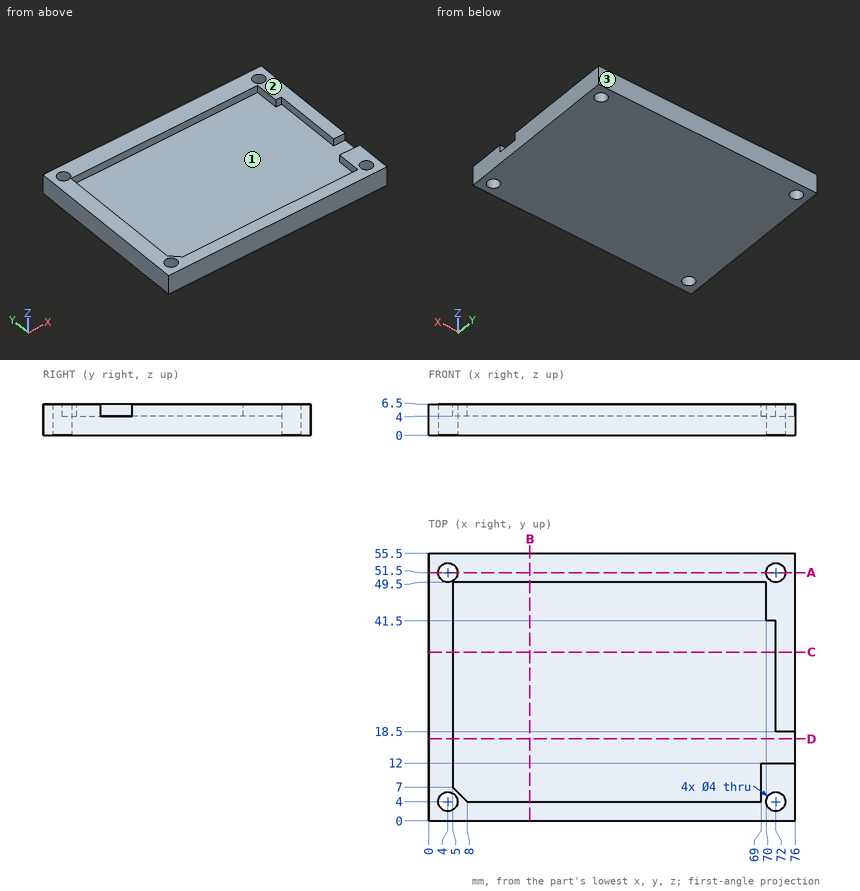
Could you check a few things on this drawing? It's one solid part, dimensions in mm from its lowest x, y, z. Give positions to 0.01 mm unless a question says otherwise; leave off trailing zeros. Write each loop counter-clockwise with the first axis right and the second up, starting at its lowest first coordinate (ties: lowest second). Pieces come first, ordered by that corner, then holes. Notation, with made-up numbers: M -26.75,-1 L -16.75,-1 A37 cw -16.75,35 Z; hole C 87,48 d1. An arc over 180 degrees is marked long. Put each result on its own line as item: value. Start each with the question number.
Item 1: If we section it at C-C, the plane y = 35: Write out the boundary of the cut face in (x, z).
Item 2: If we section it at D-D, the plane y = 17: Write out the boundary of the cut face in (x, z).
Item 3: Will this pin go through, and if not, where does the flat tip stop? pin 1 (5 mm diameter, centred on x = 20, y = 30, fed in from +Z).
Item 4: If we section it at A-A, the plane y = 51.5: Write out the boundary of the cut face in (x, z), then the cut area to 3 significant figures.
Item 5: I need wall thicknesses on L1, parallel to Y at x = 72, z = 1.75; L2, parallel to Y at x = 58, z = 5.25; L3, parallel to X at y = 3, z = 3. Which ranges of each line are inside material? Lowest first, please. Write a range as from..to.
Item 6: If we section it at B-B, the plane x = 21: Write out the boundary of the cut face in (y, z).
Item 7: Thinking about a two-plate mould opening in Y: for the marked faces 1, 2 and 3, which applies, +Y half, -Y half, draft (parallel to the pull), parting line (faces both ways), or undercut?
Values:
1. outline: M 0,0 L 76,0 L 76,6.5 L 72,6.5 L 72,4 L 5,4 L 5,6.5 L 0,6.5 Z
2. outline: M 0,0 L 76,0 L 76,4 L 5,4 L 5,6.5 L 0,6.5 Z
3. pin 1: z = 4
4. outline: M 0,0 L 2,0 L 2,6.5 L 0,6.5 Z; M 6,0 L 70,0 L 70,6.5 L 6,6.5 Z; M 74,0 L 76,0 L 76,6.5 L 74,6.5 Z
4. area: 442 mm²
5. L1: 0..2, 6..49.5, 53.5..55.5
5. L2: 0..4, 49.5..55.5
5. L3: 0..2.27, 5.73..70.27, 73.73..76
6. outline: M 0,0 L 55.5,0 L 55.5,6.5 L 49.5,6.5 L 49.5,4 L 4,4 L 4,6.5 L 0,6.5 Z
7. face 1: undercut
7. face 2: draft
7. face 3: +Y half
